Can you work these out from the model? Positions are in its coordinate system, mm. A direction names the side the tool comes from. Round coordinates to 2 decimals unless told otherwise and drop trailing zeros. Loops run counter-clockwise (first coordinate to the right, second up) from the corner with the lowest first, then second, coordinate; pieces in that order, holes last. Notation, with made-up numbers: M -12.75,44.5 L 3.25,44.5 A19 ccw 3.25,67.5 Z; hole C -27.75,-24.5 d9. An arc over 180 degrees is marked long. Return JSON: item names as keys, results as strings.
```python
from build123d import *

# Parameters (mm, degrees)
F0_R            = 266.7
F0_R_2          = 247.65
F1_DEPTH        = 635
F2_R            = 266.7
F3_DEPTH        = 50.8
F4_R            = 25.4
F5_R            = 38.1
F7_DEPTH        = 50.8
F7_COPIES_COUNT = 8
F8_R            = 31.75
F9_DEPTH        = 50.8


# Not quite as in the source:
# - a pattern or mirror of a feature is missing from the dataset's text; its kind, count and spacing are read off the source's solid
# - a feature names something its author has since deleted; it is built from what else it names


with BuildPart() as f1:
    # F0 (on Top) → F1 (new body)
    with BuildSketch(Plane.XY):
        Circle(F0_R)
        Circle(F0_R_2, mode=Mode.SUBTRACT)
    extrude(amount=F1_DEPTH)

    # F2 (on face) → F3 (join)
    with BuildSketch(Plane(origin=(0, 0, 0), x_dir=(1, 0, 0), z_dir=(0, 0, -1))):
        Circle(F2_R)
    extrude(amount=F3_DEPTH)

    # F4
    f4_edges = [f1.edges().sort_by_distance(p)[0] for p in [
        (-266.7, 0, -50.8),
    ]]
    fillet(f4_edges, radius=F4_R)

    # F5 (on face) → F7 (cut, through all)
    with BuildSketch(Plane(origin=(0, 0, -50.8), x_dir=(1, 0, 0), z_dir=(0, 0, -1))):
        with Locations((-177.8, 0)):
            Circle(F5_R)
    f7 = extrude(amount=-F7_DEPTH, mode=Mode.SUBTRACT)

    # F7_copies: F7 ×8 about axis
    f7_copies_axis = Axis((0, 0, 0), (0, 0, 1))
    for i in range(1, F7_COPIES_COUNT):
        add(f7.rotate(f7_copies_axis, i * 360 / F7_COPIES_COUNT), mode=Mode.SUBTRACT)

    # F8 (on face) → F9 (cut, through all)
    with BuildSketch(Plane(origin=(0, 0, -50.8), x_dir=(1, 0, 0), z_dir=(0, 0, -1))):
        with Locations((0, 66.04)):
            Circle(F8_R)
        with Locations((66.04, 0)):
            Circle(F8_R)
        with Locations((-66.04, 0)):
            Circle(F8_R)
        with Locations((0, -66.04)):
            Circle(F8_R)
    extrude(amount=-F9_DEPTH, mode=Mode.SUBTRACT)


solid = f1.part
```
Q1. Thinking about a two-plate mould opening in X: for faces 3 (the cylindrical face through (254.384, -80.109, 309.423)), 4 (the cylindrical face through (111.2, 90.5, -25.8)), 5 (the flat face through (-3, -3, -50.8)), 6 (the cylindrical face through (141.46, 11.44, -25.76)), which applies, pulls with the +X half, pulls with the -X half, needs draft (parallel to the pull), parting line crosses it, or undercut?
Results:
{"face 3": "parting line crosses it", "face 4": "undercut", "face 5": "needs draft", "face 6": "undercut"}
Q2. On a 3-axis mill with a long thin cutter (end or side, diameter ignored), from which of +Z, -Z, +X, -X, +Y, -Y can I reach the whole of each face in a straight line? I mean faces 1 (the flat face through (78, -236, 635)), 2 (the flat face through (-3, -3, 0)). Say none if no direction works.
Results:
{"face 1": "+Z, +X, -X, +Y, -Y", "face 2": "+Z"}
Q3. If I drill on line 1 along Z through (x, y) = (55, 194.5); line 2 along X through (y, z) = (72, 269); line 3 along Y through (x, z) = (-80.5, -5), over which ranges is the centre line in solid material (lowest first)?
Results:
{"line 1": "z = -50.8 to 0", "line 2": "x = -256.8 to -236.95, 236.95 to 256.8", "line 3": "y = -254.26 to -28.27, 28.27 to 254.26"}
Q4. I'm going to push flat-ended pins straight in: pin 1 Ø1 at (y, z) = (-193.5, 405.5) entering from -X; pin 2 Ø5 at (x, y) = (-94, -200) entering from +Z; pin 3 Ø5 at (x, z) = (-36, 37) entering from +Y. Where does each tip first touch, or does it pass through?
Results:
{"pin 1": "stops at x = -184.06", "pin 2": "stops at z = 0", "pin 3": "stops at y = 264.59"}
Q5. Suppose I cut it at A-A, the plane y = 0. Please give me the cut outline in (x, z), plus the area to 3 significant figures.
Results:
{"outline": "M -266.7,-25.4 A25.4 ccw -241.3,-50.8 L -215.9,-50.8 L -215.9,0 L -247.65,0 L -247.65,635 L -266.7,635 Z; M -139.7,-50.8 L -97.79,-50.8 L -97.79,0 L -139.7,0 Z; M -34.29,-50.8 L 34.29,-50.8 L 34.29,0 L -34.29,0 Z; M 97.79,-50.8 L 139.7,-50.8 L 139.7,0 L 97.79,0 Z; M 215.9,-50.8 L 241.3,-50.8 A25.4 ccw 266.7,-25.4 L 266.7,635 L 247.65,635 L 247.65,0 L 215.9,0 Z", "area": "36,800 mm2"}
Q6. Suppose I cut it at C-C, the plane z = 30.5. Please give me the cut outline in (x, y), plus the area to 3 significant figures.
Results:
{"outline": "C 0,0 d533.4; hole C 0,0 d495.3", "area": "30,800 mm2"}
